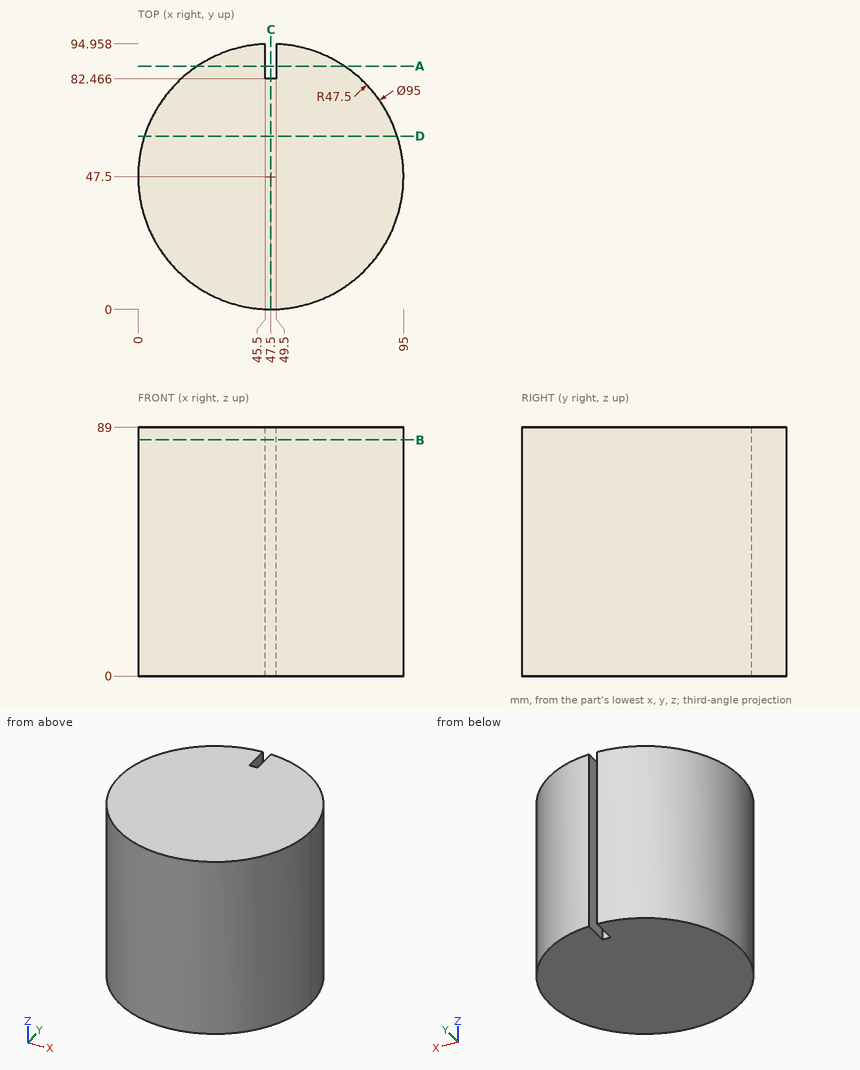
Verification items for this drawing (mm, ordinates from the low corner). Coordinates: 2 decimals unless noted, no trailing zeros. Loops run counter-clockwise (first coordinate to the right, second up) from the corner with the lowest first, then second, coordinate; pieces in that order, holes last. Notation, with made-up numbers: (27.25, -7) - (56.25, -7) arc R16 cw to (56.25, 20) - close; hole circle Ø4 at (-27.75, 67.25). An arc over 180 degrees is marked (long way). Use one line per item in the form item = value. Start each with the question number.
Item 1: Thickness scan on probe 1 along Y at (x, z) = (46, 70.5) (1 decimal); probe 2 along X at (y, z) = (90, 73.5) (1 decimal); probe 3 along X at (y, z) = (88, 73.5). Record the ranges inside material, lowest first.
Item 2: Gauge pin test, flat ends, axial feed: pin 1 (13.5 mm diameter, centred on y = 86.5, z = 28.5, fed in from -X) (1 decimal); pin 2 (2 mm diameter, centred on x = 51, z = 41, fed in from -Y); pin 3 (6 mm diameter, centred on x = 80.5, y = 81.5, fed in from -Z); pin 4 (1 mm diameter, centred on x = 46, z = 75.5, fed in from -Y). Record the tip position at first contact, or that the pin passes through.
Item 3: Section check D-D, the plane y = 62. Enter the section's corners in (x, z).
Item 4: Section check A-A, the plane y = 87. Enter the section's corners in (x, z).
Item 5: Section check B-B, the plane z = 84.5. Enter the section's corners in (x, y) (1 decimal).
Item 6: Section check C-C, the plane x = 47.5. Enter the section's corners in (y, z) (1 decimal).
Computed:
q1.probe_1 = 0 to 82.5
q1.probe_2 = 26.3 to 45.5, 49.5 to 68.7
q1.probe_3 = 22.68 to 45.5, 49.5 to 72.32
q2.pin_1 = 12.6
q2.pin_2 = 0.07
q2.pin_3 = 0
q2.pin_4 = 0.01
q3.outline = (2.27, 0) - (92.73, 0) - (92.73, 89) - (2.27, 89) - close
q4.outline = (21.12, 0) - (45.5, 0) - (45.5, 89) - (21.12, 89) - close; (49.5, 0) - (73.88, 0) - (73.88, 89) - (49.5, 89) - close
q5.outline = (45.5, 82.5) - (45.5, 95) arc R47.5 ccw (long way) to (49.5, 95) - (49.5, 82.5) - close
q6.outline = (0, 0) - (82.5, 0) - (82.5, 89) - (0, 89) - close
